Build history of the part. All positions in model axes, mm. A direction names the side the tool comes from. Give positions to 0.01 mm unless a question says otherwise; leave off trailing zeros. Order: outer loops, then holes, each group sorted by start corner. A loop starts at its lowest first (then second) coordinate and runs counter-clockwise, first axis right, second up. Notation, with made-up numbers: M 82,66.25 L 96,66.25 A25 cw 96,99.25 Z; hole C -21,78.25 d9. An arc over 180 degrees is marked long. One line per item, written item: value.
Autodesk Inventor part; units mm, degrees
ref_plane "Work Plane1" through (0, 0, 45) normal (0, 0, 1) x (1, 0, 0)
ref_plane "YZ Plane" through (0, 0, 0) normal (1, 0, 0) x (0, 1, 0)
ref_plane "XZ Plane" through (0, 0, 0) normal (0, 1, 0) x (-1, 0, 0)
sketch "Sketch1" plane through (0, 0, 0) normal (0, 1, 0) x (-1, 0, 0)
  line L0 (30, 45) -> (-30, 45)
  line L1 (-30, 45) -> (-30, -45)
  line L2 (-30, -45) -> (30, -45)
  line L3 (30, -45) -> (30, 45)
  line L4 (30, 45) -> (-30, -45) construction
  line L5 (-30, 45) -> (30, -45) construction
  point P0 (0, 0)
  dimension "d0" = 60
  dimension "d1" = 90
extrude "Extrusion1" add sketch "Sketch1" along normal blind 10
ref_plane "Work Plane1" through (0, 0, 45) normal (0, 0, 1) x (1, 0, 0)
sketch "Sketch4" plane through (0, 0, 45) normal (0, 0, 1) x (1, 0, 0)
  line L0 (-30, 10) -> (30, 10)
  line L1 (0, 10) -> (0, 30)
  line L2 (-5, 10) -> (5, 10)
  circle A0 centre (0, 30) radius 7.6
  line L3 (-13.5, 43.5) -> (13.5, 43.5)
  line L4 (13.5, 43.5) -> (13.5, 16.5)
  line L5 (13.5, 16.5) -> (-13.5, 16.5)
  line L6 (-13.5, 16.5) -> (-13.5, 43.5)
  line L7 (-13.5, 43.5) -> (13.5, 16.5) construction
  line L8 (13.5, 43.5) -> (-13.5, 16.5) construction
  line L9 (-6, 18) -> (6, 18)
  line L10 (6, 18) -> (6, 2)
  line L11 (6, 2) -> (-6, 2)
  line L12 (-6, 2) -> (-6, 18)
  line L13 (-6, 18) -> (6, 2) construction
  line L14 (6, 18) -> (-6, 2) construction
  point P0 (0, 0)
  point P1 (6, 16.5)
  point P2 (-6, 16.5)
  dimension "d11" = 20
  dimension "d27" = 15.2
  dimension "d28" = 27
  dimension "d29" = 27
  dimension "d30" = 12
  dimension "d31" = 16
extrude "Extrusion3" add sketch "Sketch4" against normal blind 10
fillet "Fillet2" radius 8 4 edges at (-30, 5, 45) (30, 5, 45) (30, 5, -45) (-30, 5, -45)
sketch "Sketch5" plane through (0, 10, 0) normal (0, 1, 0) x (1, 0, 0)
  circle A0 centre (0, 0) radius 10
  dimension "d20" = 20
extrude "Extrusion4" cut sketch "Sketch5" against normal blind 10
sketch "Sketch6" plane through (0, 0, 45) normal (0, 0, 1) x (1, 0, 0)
  point P0 (0, 0)
sketch "Sketch7" plane through (0, 0, 45) normal (0, 0, 1) x (1, 0, 0)
  point P0 (0, 0)
properties part number "BASE DE YUGO ESCOCES"
1) Tool access for faces 5 (the face through (-10, 16.5, 40)), 6 (the face through (6, 23, 35)), 7 (the face through (27.719, 5.07, -42.594)), 8 (the face through (13.5, 30, 40)), 9 (the face through (-30, 5, -1)): list every direction of +Z, -Z, +X, -X, +Y, -Y with a clear straight run to the whole face (end or side of a thin tool).
Check values:
face 5: +Z, -Z, -X
face 6: -Z, +X, -X, +Y
face 7: -Z, +X, +Y, -Y
face 8: +Z, -Z, +X, +Y
face 9: +Z, -Z, -X, +Y, -Y
2) Saw through at D-D, the plane y = 3.5. Write the cut outline in (x, z), then the cut area to 3 significant figures.
Check values:
outline: M -30,-37 A8 ccw -22,-45 L 22,-45 A8 ccw 30,-37 L 30,37 A8 ccw 22,45 L -22,45 A8 ccw -30,37 Z; hole C 0,0 d20
area: 5,030 mm^2
3) Saw through at A-A, the plane x = 0. Write the cut outline in (y, z).
Check values:
outline: M 0,-45 L 10,-45 L 10,-10 L 0,-10 Z; M 0,10 L 10,10 L 10,35 L 22.4,35 L 22.4,45 L 0,45 Z; M 37.6,35 L 43.5,35 L 43.5,45 L 37.6,45 Z
4) Mould opens along X. For faces 1 (the face through (6, 13, 40)), 2 (the face through (0, 0, 11)), 3 (the face through (-2.17, 5.07, 9.76)), 4 (the face through (-13.5, 30, 40)) say: released by +X, released by -X, zero draft, split by the parting line, or undercut.
Check values:
face 1: released by +X
face 2: zero draft
face 3: undercut
face 4: released by -X
5) Pin check, flat tips, straight feed: pin 1 (4 mm diameter, centred on x = 11, z = 39, fed in from -Y); pin 2 (2 mm diameter, centred on y = 14.5, z = 41.5, fed in from -X); pin 3 (21.5 mm diameter, centred on x = -0.5, y = 21.5, fed in from -Z); pin 4 (5 mm diameter, centred on y = 25.5, z = 37.5, fed in from -X). Stop position of each tip, or through.
Check values:
pin 1: y = 0
pin 2: x = -6
pin 3: z = 35
pin 4: x = -13.5
6) Drill centre lines: probe 1 along X at (y, z) = (3, 0); probe 2 along Z at (x, y) = (0, 7.75); probe 3 along Z at (x, y) = (11, 37.5). Where is each one in solid material? Low to high. Write a range as from..to.
Check values:
probe 1: -30..-10, 10..30
probe 2: -45..-10, 10..45
probe 3: 35..45
7) Saw through at B-B, the plane y = 30. Write the cut outline in (x, z).
Check values:
outline: M -13.5,35 L -7.6,35 L -7.6,45 L -13.5,45 Z; M 7.6,35 L 13.5,35 L 13.5,45 L 7.6,45 Z
8) Saw through at C-C, the plane z = 0. Write the cut outline in (x, y), then the cut area to 3 significant figures.
Check values:
outline: M -30,0 L -10,0 L -10,10 L -30,10 Z; M 10,0 L 30,0 L 30,10 L 10,10 Z
area: 400 mm^2
